Could you check a few things on this model? Use its own coordinates, in mm. A direction names the side the tool comes from. Round coordinates to 2 decimals unless told otherwise and drop trailing zeros. Loops run counter-clockwise (first coordinate to the right, second up) from the corner with the lowest first, then second, coordinate; pieces in that order, holes last. Notation, with made-up numbers: (-38.75, 33.5) -> (-27.75, 33.5) arc R26 cw to (-27.75, 64.5) -> close; hole circle Ø10 at (74, 45). An arc over 180 degrees is marked (long way). Put each result on its own line as item: value. Start each with the question number.
1. I'm going to push flat-ended pins straight in: P1, Ø3, axis at x = 41.656, z = -38.1, coming from the +Y side; P2, Ø5, axis at x = 80, z = -60, coming from the +Y side; P3, Ø1.9, axis at y = -4.5, z = -68, coming from the -X side; P4, Ø4, axis at x = 70.5, y = -2, coming from the +Z side. Where does each tip first touch, or does it pass through?
2. Which directions (+Z, -Z, +X, -X, +Y, -Y) give clear straight access to the entire face, cutting with the end or side of a thin tool? Please do faces 1 (the flat face through (117, -3, -53.34)), 2 (the flat face through (117, 34.29, -64)), 3 (the flat face through (45, -3, -12.7)), 4 (the flat face through (91.44, -3, -67)), 5 (the flat face through (117, 17, -17.78)).
3. I need wall thicknesses on line 1 (X direction, y = -4, z = -38.1); line 2 (Z direction, x = 114.5, y = 10.5); line 3 (X direction, y = 11.5, z = -12). Which ranges of each line are inside material? Lowest first, please. Write a range as [from, to].
4. Imagine slicing it at B-B, the plane z = -38.1. Please give me the cut outline in (x, y).
5. Imagine slicing it at C-C, the plane x = 110.49. Please give me the cut outline in (y, z), and give its area (3 significant figures).
6. Imagine slicing it at A-A, the plane x = 25.4. Please give me the cut outline in (y, z), and give its area (3 significant figures).
7. If we mould it in two halves opening along X, with no side actions, what happens to faces 6 (the cylindrical face through (109.24, 13.69, -63.62)), 7 (the flat face through (106.68, 17, -12)), 8 (the cylindrical face through (44.035, -3.219, -38.205)), 9 (the flat face through (127, 14, -63))? For each: pulls with the +X half, pulls with the -X half, needs draft (parallel to the pull), parting line crosses it, or undercut.
8. Imagine slicing it at D-D, the plane y = 19.5. Please give me the cut outline in (x, z) (3 decimals).
```python
from build123d import *

# Parameters (mm, degrees)
BOSS_EXTRUDE3_DEPTH          = 6.35
SKETCH4_W                    = 20.32
SKETCH4_H                    = 11.43
BOSS_EXTRUDE4_DEPTH          = 34.29
SKETCH5_W                    = 19.05
SKETCH5_H                    = 30.48
CUT_EXTRUDE1_DEPTH           = 12.7
F_3_16_0_1875_DOWEL_HOLE4_D  = 4.7625
F_1_4_0_2500_DOWEL_HOLE1_D   = 6.35
F_36_0_1065_DIAMETER_HOLE1_D = 2.7051
F_6_32_TAPPED_HOLE1_D        = 2.7051


with BuildPart() as part:
    # Sketch2 → Boss-Extrude3 (new body)
    with BuildSketch(Plane(origin=(0, 0, 0), x_dir=(1, 0, 0), z_dir=(0, 1, 0))):
        Polygon((91.44, 6.35), (127, 6.35), (127, 69.85), (91.44, 69.85), (91.44, 63.5), (0, 63.5), (0, 12.7), (91.44, 12.7), align=None)
    extrude(amount=-BOSS_EXTRUDE3_DEPTH)

    # Sketch4 → Boss-Extrude4 (add)
    with BuildSketch(Plane(origin=(0, 0, 0), x_dir=(1, 0, 0), z_dir=(0, 1, 0))):
        with Locations((116.84, 64.135)):
            Rectangle(SKETCH4_W, SKETCH4_H)
        with Locations((116.84, 12.065)):
            Rectangle(SKETCH4_W, SKETCH4_H)
    extrude(amount=BOSS_EXTRUDE4_DEPTH)

    # Sketch5 → Cut-Extrude1 (cut)
    with BuildSketch(Plane(origin=(0, 0, 0), x_dir=(1, 0, 0), z_dir=(0, 1, 0))):
        with Locations((117.475, 38.1)):
            Rectangle(SKETCH5_W, SKETCH5_H)
    extrude(amount=-CUT_EXTRUDE1_DEPTH, mode=Mode.SUBTRACT)

    # 3/16 (0.1875) Dowel Hole4 (through all)
    with Locations(Plane(origin=(0, 0, 0), x_dir=(1, 0, 0), z_dir=(0, 1, 0))):
        with Locations((41.656, 38.1)):
            Hole(F_3_16_0_1875_DOWEL_HOLE4_D / 2)

    # 1/4 (0.2500) Dowel Hole1 (through all)
    with Locations(Plane(origin=(0, 34.29, 0), x_dir=(1, 0, 0), z_dir=(0, 1, 0))):
        with Locations((121.92, 12.065)):
            Hole(F_1_4_0_2500_DOWEL_HOLE1_D / 2)

    # #36 (0.1065) Diameter Hole1 (through all)
    with Locations(Plane(origin=(0, 0, 0), x_dir=(1, 0, 0), z_dir=(0, 1, 0))):
        with Locations((25.4, 38.1), (79.375, 38.1)):
            Hole(F_36_0_1065_DIAMETER_HOLE1_D / 2)

    # #6-32 Tapped Hole1 (through all)
    with Locations(Plane(origin=(0, 34.29, 0), x_dir=(1, 0, 0), z_dir=(0, 1, 0))):
        with Locations((123.19, 64.135), (110.49, 64.135)):
            Hole(F_6_32_TAPPED_HOLE1_D / 2)


solid = part.part
```
Entries:
1. P1: through
1. P2: y = 0
1. P3: x = 91.44
1. P4: z = -12.7
2. face 1: +X, +Y, -Y
2. face 2: +Z, -Z, +X, -X, +Y
2. face 3: +Z, -X, +Y, -Y
2. face 4: -Z, -X, +Y, -Y
2. face 5: +X, -X, +Y
3. line 1: [0, 24.05], [26.75, 39.27], [44.04, 78.02], [80.73, 107.95]
3. line 2: [-69.85, -58.42], [-17.78, -6.35]
3. line 3: [106.68, 118.75], [125.09, 127]
4. outline: (0, -6.35) -> (24.05, -6.35) -> (24.05, 0) -> (0, 0) -> close; (26.75, -6.35) -> (39.27, -6.35) -> (39.27, 0) -> (26.75, 0) -> close; (44.04, -6.35) -> (78.02, -6.35) -> (78.02, 0) -> (44.04, 0) -> close; (80.73, -6.35) -> (107.95, -6.35) -> (107.95, 0) -> (80.73, 0) -> close
5. outline: (-6.35, -69.85) -> (34.29, -69.85) -> (34.29, -65.49) -> (-6.35, -65.49) -> close; (-6.35, -62.78) -> (34.29, -62.78) -> (34.29, -58.42) -> (0, -58.42) -> (0, -53.34) -> (-6.35, -53.34) -> close; (-6.35, -22.86) -> (0, -22.86) -> (0, -17.78) -> (34.29, -17.78) -> (34.29, -6.35) -> (-6.35, -6.35) -> close
5. area: 884 mm^2
6. outline: (-6.35, -63.5) -> (0, -63.5) -> (0, -39.45) -> (-6.35, -39.45) -> close; (-6.35, -36.75) -> (0, -36.75) -> (0, -12.7) -> (-6.35, -12.7) -> close
6. area: 305 mm^2
7. face 6: undercut
7. face 7: pulls with the -X half
7. face 8: undercut
7. face 9: pulls with the +X half
8. outline: (106.68, -69.85) -> (127, -69.85) -> (127, -58.42) -> (106.68, -58.42) -> close; (106.68, -17.78) -> (127, -17.78) -> (127, -6.35) -> (106.68, -6.35) -> close; hole circle Ø2.705 at (110.49, -64.135); hole circle Ø6.35 at (121.92, -12.065); hole circle Ø2.705 at (123.19, -64.135)
